```python
from build123d import *

# Parameters (mm, degrees)
SKETCH006_W           = 3
SKETCH006_H           = 3
PAD001_DEPTH          = 1.25
CHAMFER_SIZE          = 0.5
POLARPATTERN001_COUNT = 22


with BuildPart() as part:
    # Sketch006 → Pad001 (new body)
    with BuildSketch(Plane.YZ.offset(11.25)):
        with Locations((0, -4.5)):
            Rectangle(SKETCH006_W, SKETCH006_H)
    extrude(amount=-PAD001_DEPTH)

    # Chamfer
    chamfer_edges = [part.edges().sort_by_distance(p)[0] for p in [
        (11.25, 1.5, -4.5),
        (11.25, 0, -3),
        (11.25, -1.5, -4.5),
        (11.25, 0, -6),
    ]]
    chamfer(chamfer_edges, length=CHAMFER_SIZE)

    # PolarPattern001: part ×22 about axis
    polarpattern001_axis = Axis((0, 0, 0), (0, 0, 1))


with BuildPart() as part_1:
    add(part.part)
    for i in range(1, POLARPATTERN001_COUNT):
        add(part.part.rotate(polarpattern001_axis, i * 360 / POLARPATTERN001_COUNT))


solid = part_1.part
```
Read the model definition and answer for the solid it produces. Units are mm, in the model's axes. A direction names the side the tool comes from. Give positions to 0.01 mm unless a question says otherwise; leave off trailing zeros. Order: outer loops, then holes, each group sorted by start corner. A loop starts at its lowest first (then second) coordinate and runs counter-clockwise, first axis right, second up.
(1) Given pin 1 (1.5 mm diameter, centred on x = -8, z = -4.5, fed in from +Y), flat-ended and moving along its own axis, determine where the tip first touches the part or whether it passes through.
(2) For faces 4 (the flat face through (-10, 0, -4)), 5 (the flat face through (-10.55, 3.12, -5.75)), determine the directions among +Z, -Z, +X, -X, +Y, -Y from which every point of the face is accessible in a straight line to the end or side of a thin tool.
(3) Straight lines are drawn through the part: L1, parallel to X at y = -3.5, z = -4; L2, parallel to Y at x = 2, z = -4.1; L3, parallel to X at y = 3, z = -5.8. For each, find the intervals that lie inside material, in ascending order.
(4) For a pull along Y with two mould halves and no side action, classify faces 1 (the flat face through (8.423, 5.389, -4.479)), 2 (the flat face through (9.245, -5.967, -5.747)), 3 (the flat face through (10.798, 3.156, -4.486)) as released by +Y, released by -Y, zero draft, split by the parting line, or undercut.
(5) Find section B-B (y = -3.5). Give the vertices of the cut face in (x, z).
(6) Find section A-A (x = 2.25). Give the vertices of the cut face in (y, z).
Result sheet:
1. pin 1: stops at y = 8.6
2. face 4: +Z, -Z
2. face 5: -Z, -X, +Y
3. L1: x = -10.7 to -9.39, 9.39 to 10.7
3. L2: y = -11.08 to -9.82, 9.82 to 11.08
3. L3: x = -10.53 to -9.54, 9.54 to 10.53
4. face 1: undercut
4. face 2: released by -Y
4. face 3: released by +Y
5. outline: (-10.7, -5.5) - (-10.18, -6) - (-9.39, -6) - (-9.39, -3) - (-10.18, -3) - (-10.7, -3.5) - close; (9.39, -6) - (10.18, -6) - (10.7, -5.5) - (10.7, -3.5) - (10.18, -3) - (9.39, -3) - close
6. outline: (-11.04, -5.5) - (-10.54, -6) - (-9.78, -6) - (-9.78, -3) - (-10.54, -3) - (-11.04, -3.5) - close; (9.78, -6) - (10.54, -6) - (11.04, -5.5) - (11.04, -3.5) - (10.54, -3) - (9.78, -3) - close
